from build123d import *

# Parameters (mm, degrees)
SKETCH1_W          = 16.5
SKETCH1_H          = 1.5
CHAMFER1_SIZE      = 0.1
SKETCH2_W          = 43.906364016
SKETCH2_H          = 2
CUT_EXTRUDE1_DEPTH = 15.579523312
CHAMFER2_SIZE      = 0.3


with BuildPart() as part:
    # Sketch1 → Revolve1 (revolve)
    with BuildSketch(Plane.XY, mode=Mode.PRIVATE) as revolve1_sk:
        with Locations((0, 7.75)):
            Rectangle(SKETCH1_W, SKETCH1_H)
    revolve(revolve1_sk.sketch.rotate(Axis((0, 0, 0), (1, 0, 0)), 90), axis=Axis((0, 0, 0), (1, 0, 0)))

    # Chamfer1
    chamfer1_edges = [part.edges().sort_by_distance(p)[0] for p in [
        (-8.25, 0, -7),
        (8.25, 0, -7),
        (8.25, 0, -8.5),
        (-8.25, 0, -8.5),
    ]]
    chamfer(chamfer1_edges, length=CHAMFER1_SIZE)

    # Sketch2 → Cut-Extrude1 (cut, through all)
    with BuildSketch(Plane.XY):
        Rectangle(SKETCH2_W, SKETCH2_H)
    extrude(amount=-CUT_EXTRUDE1_DEPTH, mode=Mode.SUBTRACT)

    # Chamfer2
    # the kernel refuses this chamfer: 0.354238868, 0.3, 0.270099322 mm, written as the material it takes off along each edge
    with BuildSketch(Plane(origin=(8.25, 1, -6.257719812), x_dir=(-1, 0, 0), z_dir=(0, 0, -1)), Plane(origin=(-8.25, 1, -9.111768681), x_dir=(1, 0, 0), z_dir=(0, 0, 1)), Plane(origin=(-8.25, -1, -6.257719812), x_dir=(1, 0, 0), z_dir=(0, 0, -1))) as chamfer2_piece_1:
        Polygon((CHAMFER2_SIZE, 0), (0, CHAMFER2_SIZE), (0, 0), align=None)
    extrude(amount=2.854048869, mode=Mode.SUBTRACT)
    with BuildSketch(Plane(origin=(8.25, -1, -9.111768681), x_dir=(0, -1, 0), z_dir=(0, 0, 1))) as chamfer2_piece_2:
        Polygon((CHAMFER2_SIZE, 0), (0, -CHAMFER2_SIZE), (0, 0), align=None)
    extrude(amount=2.854048869, mode=Mode.SUBTRACT)
    with BuildSketch(Plane(origin=(8.921504896, -1, -8.440971508), x_dir=(0, 0, 1), z_dir=(-1, 0, 0))) as chamfer2_piece_3:
        with BuildLine():
            Line((CHAMFER2_SIZE, 0), (0.035547132, -0.264452868))
            ThreePointArc((0.035547132, -0.264452868), (0.01722122, -0.135971426), (0, 0))
            Line((0, 0), (CHAMFER2_SIZE, 0))
        make_face()
    extrude(amount=17.843009793, mode=Mode.SUBTRACT)
    with BuildSketch(Plane(origin=(8.921504896, 1, -8.440971508), x_dir=(0, 0, 1), z_dir=(-1, 0, 0))) as chamfer2_piece_4:
        with BuildLine():
            Line((CHAMFER2_SIZE, 0), (0.035547132, 0.264452868))
            ThreePointArc((0.035547132, 0.264452868), (0.01722122, 0.135971426), (0, 0))
            Line((0, 0), (CHAMFER2_SIZE, 0))
        make_face()
    extrude(amount=17.843009793, mode=Mode.SUBTRACT)
    with BuildSketch(Plane(origin=(-9.097260331, -1, -6.92820323), x_dir=(0, 0, -1), z_dir=(1, 0, 0))) as chamfer2_piece_5:
        with BuildLine():
            Line((CHAMFER2_SIZE, 0), (-0.061980996, -0.361980996))
            ThreePointArc((-0.061980996, -0.361980996), (-0.029595535, -0.187102296), (0, 0))
            Line((0, 0), (CHAMFER2_SIZE, 0))
        make_face()
    extrude(amount=18.194520662, mode=Mode.SUBTRACT)
    with BuildSketch(Plane(origin=(-9.097260331, 1, -6.92820323), x_dir=(0, 0.9856552884232092, 0.16877100581367702), z_dir=(1, 0, 0))) as chamfer2_piece_6:
        with BuildLine():
            Line((0.367249078, 0), (-CHAMFER2_SIZE * 0.168771005814, -CHAMFER2_SIZE * 0.985655288423))
            Line((-CHAMFER2_SIZE * 0.168771005814, -CHAMFER2_SIZE * 0.985655288423), (0, 0))
            ThreePointArc((0, 0), (0.189413236, -0.002406447), (0.367249078, 0))
        make_face()
    extrude(amount=18.194520662, mode=Mode.SUBTRACT)


solid = part.part
Geometry check sheet. Reference: the model listing, model coordinates, mm. A direction names the side the tool comes from. Give positions to 0.01 mm unless a question says otherwise; leave off trailing zeros. Loops run counter-clockwise (first coordinate to the right, second up) from the corner with the lowest first, then second, coordinate; pieces in that order, holes last. Notation, with made-up numbers: M -0.75,-6 L 52.25,-6 A16 cw 52.25,0 Z; hole C -10.5,80 d8. An arc over 180 degrees is marked long. Answer as a JSON object with one key per item and string values. Group by question number.
Item 1: Sectioned sample at B-B on x = 2. Record the boundary of the cut face in (y, z), plus the area to 3 significant figures.
Item 2: Mould release check, pull along Y, two halves, no side actions. Record for faces 1 (the flat face through (8.25, -2, 7)), 2 (the cylindrical face through (0.114, 0.356, 8.493)), 3 (the cylindrical face through (0, 0, 7)): pulls with the +Y half, pulls with the -Y half, needs draft (parallel to the pull), parting line crosses it, or undercut.
Item 3: Sectioned sample at A-A on z = 0. Record the boundary of the cut face in (x, y), plus the area to 3 significant figures.
Item 4: Access from +Z, -Z, +X, -X, +Y, -Y to the whole of each face (thin tool, end or side, straight path). Record for faces 4 (the flat face through (-8.25, -2, 7)), 5 (the flat face through (-0.1, -1, -7.7)).
Item 5: Sectioned sample at C-C on y = 0. Record the boundary of the cut face in (x, z).
Item 6: Material ranges on L1, parallel to Y at x = -2.5, z = 0; L2, parallel to Y at x = -3.75, z = 5.5; L3, parallel to Z at x = 7, y = 3.5, recorded low to high.
Item 7: Gauge pin test, flat ends, axial feed: pin 1 (5 mm diameter, centred on x = -0.5, y = 5, fed in from +Z); pin 2 (5 mm diameter, centred on x = -5.5, y = 4, fed in from -Z); pin 3 (0.5 mm diameter, centred on x = 3, z = -7.5, fed in from +Y). Record the tip position at first contact, or that the pin passes through.
Findings below:
{
 "1": {"outline": "M -1.36,-6.87 A7 cw long 1.36,-6.87 L 1,-7.23 L 1,-8.14 L 1.26,-8.41 A8.5 ccw long -1.26,-8.41 L -1,-8.14 L -1,-7.23 Z", "area": "69.8 mm2"},
 "2": {"face 1": "needs draft", "face 2": "parting line crosses it", "face 3": "undercut"},
 "3": {"outline": "M -8.25,-8.4 L -8.15,-8.5 L 8.15,-8.5 L 8.25,-8.4 L 8.25,-7.1 L 8.15,-7 L -8.15,-7 L -8.25,-7.1 Z; M -8.25,7.1 L -8.15,7 L 8.15,7 L 8.25,7.1 L 8.25,8.4 L 8.15,8.5 L -8.15,8.5 L -8.25,8.4 Z", "area": "49.5 mm2"},
 "4": {"face 4": "+Z, -Z, -X, +Y, -Y", "face 5": "-Z, +X, -X"},
 "5": {"outline": "M -8.25,7.1 L -8.15,7 L 8.15,7 L 8.25,7.1 L 8.25,8.4 L 8.15,8.5 L -8.15,8.5 L -8.25,8.4 Z"},
 "6": {"L1": "-8.5 to -7, 7 to 8.5", "L2": "-6.48 to -4.33, 4.33 to 6.48", "L3": "-7.75 to -6.06, 6.06 to 7.75"},
 "7": {"pin 1": "z = 8.12", "pin 2": "z = -8.37", "pin 3": "y = 4.44"}
}
